from build123d import *

# Parameters (mm, degrees)
F0_W     = 50
F0_H     = 20
F1_DEPTH = 60
F2_W     = 9
F2_H     = 25.2990102768
F2_W_2   = 32
F3_DEPTH = 25
F4_R     = 2.5
F5_DEPTH = 60
F7_DEPTH = 25
F9_DEPTH = 25


with BuildPart() as f1:
    # F0 (on Top) → F1 (new body)
    with BuildSketch(Plane.XY):
        with Locations((3.2706648111, 10)):
            Rectangle(F0_W, F0_H)
    extrude(amount=F1_DEPTH)

    # F2 (on face) → F3 (cut)
    with BuildSketch(Plane.XZ):
        with Locations((-17.2293351889, 47.3504948616)):
            Rectangle(F2_W, F2_H)
        with Locations((23.7706648111, 47.3504948616)):
            Rectangle(F2_W, F2_H)
        with Locations((3.2706648111, 47.3504948616)):
            Rectangle(F2_W_2, F2_H)
    extrude(amount=-F3_DEPTH, mode=Mode.SUBTRACT)

    # F4 (on face) → F5 (cut)
    with BuildSketch(Plane(origin=(0, 0, 0), x_dir=(1, 0, 0), z_dir=(0, 0, -1))):
        with Locations((23.7706648111, -10)):
            Circle(F4_R)
        with Locations((-17.2293351889, -10)):
            Circle(F4_R)
    extrude(amount=-F5_DEPTH, mode=Mode.SUBTRACT)

    # F6 (on face) → F7 (cut)
    with BuildSketch(Plane(origin=(0, 20, 0), x_dir=(-1, 0, 0), z_dir=(0, 1, 0))):
        with BuildLine():
            Line((-16.1088471688, 34.7009897232), (9.5675175466, 34.7009897232))
            ThreePointArc((9.5675175466, 34.7009897232), (-3.2706648111, 41.520220155), (-16.1088471688, 34.7009897232))
        make_face()
        with BuildLine():
            ThreePointArc((12.2238130515, 26.0257422924), (11.5448638087, 30.562145708), (9.5675175466, 34.7009897232))
            Line((9.5675175466, 34.7009897232), (-16.1088471688, 34.7009897232))
            ThreePointArc((-16.1088471688, 34.7009897232), (-7.8070682267, 11.2102136725), (12.2238130515, 26.0257422924))
        make_face()
    extrude(amount=-F7_DEPTH, mode=Mode.SUBTRACT)

    # F8 (on face) → F9 (cut)
    with BuildSketch(Plane(origin=(0, 20, 0), x_dir=(-1, 0, 0), z_dir=(0, 1, 0))):
        with BuildLine():
            Line((-18.7576970823, 34.7009897232), (-18.7576970823, 26.5060293604))
            ThreePointArc((-18.7576970823, 26.5060293604), (-18.0140969007, 30.7912490289), (-16.1088471688, 34.7009897232))
            Line((-16.1088471688, 34.7009897232), (-18.7576970823, 34.7009897232))
        make_face()
        with BuildLine():
            ThreePointArc((9.5675175466, 34.7009897232), (11.3354625842, 31.1968047313), (12.1661882356, 27.3608124208))
            Line((12.1661882356, 27.3608124208), (12.1661882356, 34.7009897232))
            Line((12.1661882356, 34.7009897232), (9.5675175466, 34.7009897232))
        make_face()
    extrude(amount=-F9_DEPTH, mode=Mode.SUBTRACT)


solid = f1.part
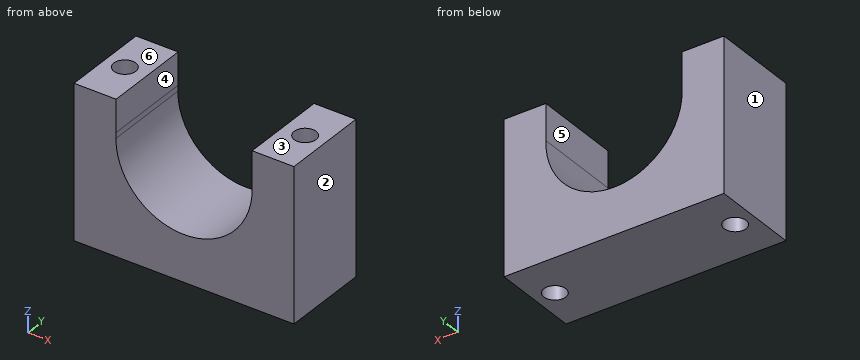
For this review, take the finished solid that the model builds, in its own axes (mm). Face numbers are marked on the shaded views. A direction names the side the tool comes from. Give positions to 0.01 mm unless a question says otherwise; leave off trailing zeros. Loops run counter-clockwise (first coordinate to the right, second up) from the corner with the lowest first, then second, coordinate; pieces in that order, holes last.
Item 1: Take a section at D-D, the plane x = -17. State the section outline as (y, z) points.
Item 2: Tool access review of the marked faces 5 and 6: name each direction out of +Z, -Z, +X, -X, +Y, -Y from which nothing blocks a thin tool from reaching the whole face with its end or side.
Item 3: Take a section at C-C, the plane y = 17. State the section outline as (x, z) points, and give its area (3 significant figures).
Item 4: Draft analysis for pull direction X (two halves, no side actions). For the marked faces 1, 2, 3 and 4, state which applies: +X half, -X half, draft (parallel to the pull), parting line (faces both ways), or undercut.
Item 5: Take a section at B-B, the plane y = 10. State the section outline as (x, z) points, and give its area (3 significant figures).
Item 6: For line 1 along X through (y, z) = (10, 8); line 2 along X through (y, z) = (10, 28); line 3 along X through (y, z) = (10.5, 33), list the stretches that pass through material, from the lowest coordinate up.
Item 7: Insertion check: pin 1 (1 mm diameter, centred on x = 3.5, y = 3, fed in from +Z). The pin has a flat end and moves straight along its axis. Give the tip position at first contact, or say it passes through.
Item 8: Take a section at A-A, the plane z = 30.5. State the section outline as (x, y) points.
Calculated:
1. outline: (0, 0) - (7.51, 0) - (7.51, 34.7) - (0, 34.7) - close; (12.49, 0) - (20, 0) - (20, 34.7) - (12.49, 34.7) - close
2. face 5: +Z, +Y, -Y
2. face 6: +Z, +X, -X, +Y, -Y
3. outline: (-21.73, 0) - (28.27, 0) - (28.27, 34.7) - (18.76, 34.7) - (18.76, 26.51) arc R15.49 cw (long way) to (-12.17, 27.36) - (-12.17, 34.7) - (-21.73, 34.7) - close
3. area: 1,090 mm2
4. face 1: -X half
4. face 2: +X half
4. face 3: draft
4. face 4: undercut
5. outline: (-21.73, 0) - (-19.73, 0) - (-19.73, 34.7) - (-21.73, 34.7) - close; (-14.73, 0) - (21.27, 0) - (21.27, 34.7) - (18.76, 34.7) - (18.76, 26.51) arc R15.49 cw (long way) to (-12.17, 27.36) - (-12.17, 34.7) - (-14.73, 34.7) - close; (26.27, 0) - (28.27, 0) - (28.27, 34.7) - (26.27, 34.7) - close
5. area: 743 mm2
6. line 1: x = -21.73 to -19.73, -14.73 to 21.27, 26.27 to 28.27
6. line 2: x = -21.73 to -19.73, -14.73 to -12.17, 18.76 to 21.27, 26.27 to 28.27
6. line 3: x = -21.73 to -19.68, -14.78 to -12.17, 18.76 to 21.32, 26.22 to 28.27
7. pin 1: stops at z = 10.55
8. outline: (-21.73, 0) - (-12.17, 0) - (-12.17, 20) - (-21.73, 20) - close; (18.76, 0) - (28.27, 0) - (28.27, 20) - (18.76, 20) - close; hole circle Ø5 at (-17.23, 10); hole circle Ø5 at (23.77, 10)
